from build123d import *

# Parameters (mm, degrees)
SKETCH1_W           = 30
SKETCH1_H           = 15
BOSS_EXTRUDE1_DEPTH = 30
CUT_EXTRUDE1_DEPTH  = 15
SKETCH4_3_R         = 7.5
CUT_EXTRUDE2_DEPTH  = 15
CUT_EXTRUDE3_START  = 35
SKETCH4_4_R         = 15
SKETCH4_4_R_2       = 7.5
CUT_EXTRUDE3_DEPTH  = 20
CUT_EXTRUDE4_START  = -15
SKETCH4_5_R         = 15
SKETCH4_5_R_2       = 7.5
CUT_EXTRUDE4_DEPTH  = 20
CUT_EXTRUDE5_START  = 10
SKETCH1_3_W         = 30
SKETCH1_3_H         = 15
CUT_EXTRUDE5_DEPTH  = 10


with BuildPart() as part:
    # Sketch1 → Boss-Extrude1 (new body)
    with BuildSketch(Plane(origin=(0, 0, 0), x_dir=(0, 0, -1), z_dir=(1, 0, 0))):
        with BuildLine():
            Line((0, -30), (-65, -30))
            Line((-65, -30), (-65, -25))
            Line((-65, -25), (-29.063054532, -7.439009429))
            ThreePointArc((-29.063054532, -7.439009429), (-27.651554679, 11.635786344), (-15, 25.980762114))
            Line((-15, 25.980762114), (-15, 50))
            Line((-15, 50), (-5, 50))
            Line((-5, 50), (-5, 19.364916731))
            ThreePointArc((-5, 19.364916731), (0, -20), (5, 19.364916731))
            Line((5, 19.364916731), (5, 50))
            Line((5, 50), (15, 50))
            Line((15, 50), (15, 25.980762114))
            ThreePointArc((15, 25.980762114), (28.977774789, -7.764571353), (0, -30))
        make_face()
        with Locations((-50, -37.5)):
            Rectangle(SKETCH1_W, SKETCH1_H)
    extrude(amount=BOSS_EXTRUDE1_DEPTH)

    # Sketch4 → Cut-Extrude1 (cut, symmetric)
    with BuildSketch(Plane.XY):
        with BuildLine():
            ThreePointArc((0, 35), (4.393398282, 45.606601718), (15, 50))
            Line((15, 50), (0, 50))
            Line((0, 50), (0, 35))
        make_face()
        with BuildLine():
            Line((30, 50), (15, 50))
            ThreePointArc((15, 50), (25.606601718, 45.606601718), (30, 35))
            Line((30, 35), (30, 50))
        make_face()
    extrude(amount=CUT_EXTRUDE1_DEPTH, both=True, mode=Mode.SUBTRACT)

    # Sketch4<3> → Cut-Extrude2 (cut, symmetric)
    with BuildSketch(Plane.XY):
        with Locations((15, 35)):
            Circle(SKETCH4_3_R)
    extrude(amount=CUT_EXTRUDE2_DEPTH, both=True, mode=Mode.SUBTRACT)

    # Sketch4<4> → Cut-Extrude3 (cut)
    with BuildSketch(Plane.XY.offset(CUT_EXTRUDE3_START)):
        with Locations((15, 35)):
            Circle(SKETCH4_4_R)
        with Locations((15, 35)):
            Circle(SKETCH4_4_R_2, mode=Mode.SUBTRACT)
    extrude(amount=-CUT_EXTRUDE3_DEPTH, mode=Mode.SUBTRACT)

    # Sketch4<5> → Cut-Extrude4 (cut)
    with BuildSketch(Plane.XY.offset(CUT_EXTRUDE4_START)):
        with Locations((15, 35)):
            Circle(SKETCH4_5_R)
        with Locations((15, 35)):
            Circle(SKETCH4_5_R_2, mode=Mode.SUBTRACT)
    extrude(amount=-CUT_EXTRUDE4_DEPTH, mode=Mode.SUBTRACT)

    # Sketch1<3> → Cut-Extrude5 (cut)
    with BuildSketch(Plane(origin=(0, 0, 0), x_dir=(0, 0, -1), z_dir=(1, 0, 0)).offset(CUT_EXTRUDE5_START)):
        with Locations((-50, -37.5)):
            Rectangle(SKETCH1_3_W, SKETCH1_3_H)
    extrude(amount=CUT_EXTRUDE5_DEPTH, mode=Mode.SUBTRACT)


solid = part.part
Work out the finished part from the listing and answer in its coordinate system (mm). A direction names the side the tool comes from. Round coordinates to 2 decimals unless told otherwise and drop trailing zeros. Write each loop counter-clockwise with the first axis right and the second up, starting at its lowest first coordinate (ties: lowest second). Pieces come first, ordered by that corner, then holes. Notation, with made-up numbers: M 3,28.25 L 37,28.25 A16 cw 37,47.25 Z; hole C 60.25,-9.75 d10. An arc over 180 degrees is marked long. Use a Markdown table: item, result.
1) The part is cut by section D-D on z = 17. Give the vertices of the cut face in (x, y), plus the area to 3 significant figures.
Taken from the geometry:
| item | result |
|---|---|
| outline | M 0,-30 L 30,-30 L 30,-10.54 L 0,-10.54 Z; M 0,10.54 L 30,10.54 L 30,24.72 L 25.92,24.72 A15 cw 4.08,24.72 L 0,24.72 Z |
| area | 938 mm2 |
2) Determine the mould class of faces 4 (the face through (14.79, -19.984, 0.809)), 5 (the face through (15, 20, -18)), 6 (the face through (30, -5, 21)) for opening direction Y: pulls with the +Y half, pulls with the -Y half, needs draft (parallel to the pull), parting line crosses it, or undercut.
Taken from the geometry:
| item | result |
|---|---|
| face 4 | undercut |
| face 5 | pulls with the +Y half |
| face 6 | needs draft |
3) Which of the six approach directions +Z, -Z, +X, -X, +Y, -Y give full straight-line access (tool end or side, diameter ignored) to faces 1 (the face through (20, -37, 50)), 2 (the face through (15, 20, 18)), 3 (the face through (11, 28, 5))?
Taken from the geometry:
| item | result |
|---|---|
| face 1 | +Z, -Z, -Y |
| face 2 | +Z, +Y |
| face 3 | +X, -X, +Y |
4) The part is cut by section A-A on z = -8. Give the vertices of the cut face in (x, y).
Taken from the geometry:
| item | result |
|---|---|
| outline | M 0,-28.91 L 30,-28.91 L 30,-18.33 L 0,-18.33 Z; M 0,18.33 L 30,18.33 L 30,35 A15 ccw 0,35 Z; hole C 15,35 d15 |
5) The part is cut by section B-B on y = 30.5. Give the vertices of the cut face in (x, z).
Taken from the geometry:
| item | result |
|---|---|
| outline | M 0,-15 L 9,-15 L 9,-5 L 0,-5 Z; M 0,5 L 9,5 L 9,15 L 0,15 Z; M 21,-15 L 30,-15 L 30,-5 L 21,-5 Z; M 21,5 L 30,5 L 30,15 L 21,15 Z |
6) The part is cut by section C-C on y = 18. Give the vertices of the cut face in (x, z), plus the area to 3 significant figures.
Taken from the geometry:
| item | result |
|---|---|
| outline | M 0,-24 L 30,-24 L 30,-8.72 L 0,-8.72 Z; M 0,8.72 L 30,8.72 L 30,24 L 0,24 Z |
| area | 917 mm2 |
7) Flat-ended cylindrical pins translate along their axes: pin 1 (1 mm diameter, centred on x = 12.5, y = -11.5, fed in from +Z); pin 2 (3 mm diameter, centred on x = 21, y = 0, fed in from +Z); pin 3 (5 mm diameter, centred on x = 5.5, y = 9, fed in from -Z); pin 4 (8 mm diameter, centred on y = -26.5, z = -19, fed in from +X). Find the tip coordinate at first contact, or state that the pin passes through.
Taken from the geometry:
| item | result |
|---|---|
| pin 1 | stops at z = 38.4 |
| pin 2 | stops at z = 30 |
| pin 3 | stops at z = -29.29 |
| pin 4 | stops at x = 30 |
8) Consider line 1 (Y direction, x = 17, z = -13.5); line 2 (Z direction, x = 8, y = 0); line 3 (Y direction, x = 15, z = 7.5). Determine where each line is inside the solid, lowest interval first. Write a range as [from, to].
Taken from the geometry:
| item | result |
|---|---|
| line 1 | y = [-26.79, -14.76], [14.76, 27.77], [42.23, 49.87] |
| line 2 | z = [-30, -20], [20, 30] |
| line 3 | y = [-30, -18.54], [18.54, 27.5], [42.5, 50] |
